Build history of the part. All positions in model axes, mm. Face numbers are marked on the shaded views. A direction names the side the tool comes from. Give positions to 0.01 mm unless a question says otherwise; leave off trailing zeros. Write each loop counter-clockwise with the first axis right and the second up, starting at its lowest first coordinate (ties: lowest second). Pieces come first, ordered by that corner, then holes. Notation, with made-up numbers: (2.5, 20) -> (10.5, 20) arc R6 ccw to (10.5, 29) -> close; hole circle Ø3 at (30, 78.25). An arc over 180 degrees is marked (long way). One line per question, with ' | ' between items. Start each with the question number.
(1) Band-saw the part on D-D, the plane z = 5. Give the cut face in (x, y), and give its area (3 significant figures).
(2) Band-saw the part on A-A, the plane z = 11.25. Give the cut face in (x, y).
(3) Pin check, flat tips, straight feed: P1, Ø8.5, axis at x = 34.5, y = 35.5, coming from the +Z side; P2, Ø16, axis at x = -11, z = 5.5, coming from the +Y side; P3, Ø1.6, axis at x = -5.5, y = 1, coming from the +Z side. Stop position of each tip, or through.
(4) Drill centre lines: probe 1 along X at (y, z) = (0.95, 11.25); probe 2 along Z at (x, y) = (30.5, 45); probe 3 along Z at (x, y) = (30, 1.6). Where is each one in solid material? Low to high. Write a range as from..to.
(5) Band-saw the part on C-C, the plane x = -24.5. Give the cut face in (y, z), and give its area (3 significant figures).
(6) Tool access for the marked faces 1 and 2: list every direction of +Z, -Z, +X, -X, +Y, -Y with a clear straight run to the whole face (end or side of a thin tool).
(7) Band-saw the part on B-B, the plane y = 10. Give the cut face in (x, z).
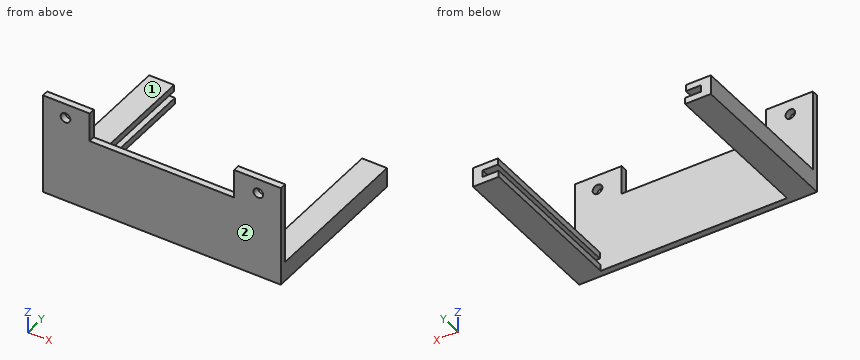
from build123d import *

# Parameters (mm, degrees)
SKETCH1_R           = 1.5
BOSS_EXTRUDE1_DEPTH = 2
BOSS_EXTRUDE2_DEPTH = 50.8


with BuildPart() as part:
    # Sketch1 → Boss-Extrude1 (new body)
    with BuildSketch(Plane(origin=(0, 0, 0), x_dir=(1, 0, 0), z_dir=(0, 1, 0))):
        Polygon((29, 15.75), (-29, 15.75), (-29, 13.75), (-34, 13.75), (-34, 11.65), (-29.25, 11.65), (-29.25, 9.65), (-37, 9.65), (-37, -15.75), (-22.5, -15.75), (-22.5, -6.75), (22.5, -6.75), (22.5, -15.75), (37, -15.75), (37, 9.65), (29.25, 9.65), (29.25, 11.65), (34, 11.65), (34, 13.75), (29, 13.75), align=None)
        with Locations((-30, -11.25)):
            Circle(SKETCH1_R, mode=Mode.SUBTRACT)
        with Locations((30, -11.25)):
            Circle(SKETCH1_R, mode=Mode.SUBTRACT)
        Polygon((-29, 13.75), (-29, 15.75), (-37, 15.75), (-37, 9.65), (-29.25, 9.65), (-29.25, 11.65), (-34, 11.65), (-34, 13.75), align=None)
        Polygon((37, 15.75), (29, 15.75), (29, 13.75), (34, 13.75), (34, 11.65), (29.25, 11.65), (29.25, 9.65), (37, 9.65), align=None)
    extrude(amount=BOSS_EXTRUDE1_DEPTH)

    # Sketch1_3 → Boss-Extrude2 (add)
    with BuildSketch(Plane(origin=(0, 0, 0), x_dir=(1, 0, 0), z_dir=(0, 1, 0))):
        Polygon((-29, 13.75), (-29, 15.75), (-37, 15.75), (-37, 9.65), (-29.25, 9.65), (-29.25, 11.65), (-34, 11.65), (-34, 13.75), align=None)
        Polygon((37, 15.75), (29, 15.75), (29, 13.75), (34, 13.75), (34, 11.65), (29.25, 11.65), (29.25, 9.65), (37, 9.65), align=None)
    extrude(amount=BOSS_EXTRUDE2_DEPTH)


solid = part.part
Results:
1) outline: (-37, 0) -> (37, 0) -> (37, 2) -> (-37, 2) -> close | area: 148 mm²
2) outline: (-37, 0) -> (-31.5, 0) -> (-31.5, 2) -> (-37, 2) -> close; (-28.5, 0) -> (-22.5, 0) -> (-22.5, 2) -> (-28.5, 2) -> close; (22.5, 0) -> (28.5, 0) -> (28.5, 2) -> (22.5, 2) -> close; (31.5, 0) -> (37, 0) -> (37, 2) -> (31.5, 2) -> close
3) P1: stops at z = -9.65 | P2: stops at y = 2 | P3: stops at z = 6.75
4) probe 1: x = -37..-31.5, -28.5..-22.5, 22.5..28.5, 31.5..37 | probe 2: z = -15.75..-13.75, -11.65..-9.65 | probe 3: z = -15.75..9.75, 12.75..15.75
5) outline: (0, -15.75) -> (2, -15.75) -> (2, 15.75) -> (0, 15.75) -> close | area: 63.0 mm²
6) face 1: +Z, +X, -X, +Y | face 2: +Z, -Z, +X, -X, -Y
7) outline: (-37, -15.75) -> (-29, -15.75) -> (-29, -13.75) -> (-34, -13.75) -> (-34, -11.65) -> (-29.25, -11.65) -> (-29.25, -9.65) -> (-37, -9.65) -> close; (29, -15.75) -> (37, -15.75) -> (37, -9.65) -> (29.25, -9.65) -> (29.25, -11.65) -> (34, -11.65) -> (34, -13.75) -> (29, -13.75) -> close
